The figure shows three views and two pictorial views of one solid part (mm, origin at its lowest corner). Answer the questions. A direction names the side the tool comes from. Give positions to 0.01 mm unless a question says otherwise; leave off trailing zeros. Write each loop counter-clockwise with the first axis right and the second up, starting at its lowest first coordinate (ties: lowest second). Pieces come first, ordered by that corner, then holes. Notation, with made-up numbers: (19, 63.25) -> (36, 63.25) arc R10 cw to (36, 73.25) -> close; hole circle Ø1 at (49.25, 23.25). An arc over 180 degrees is marked (long way). Use a Markdown table: item, result.
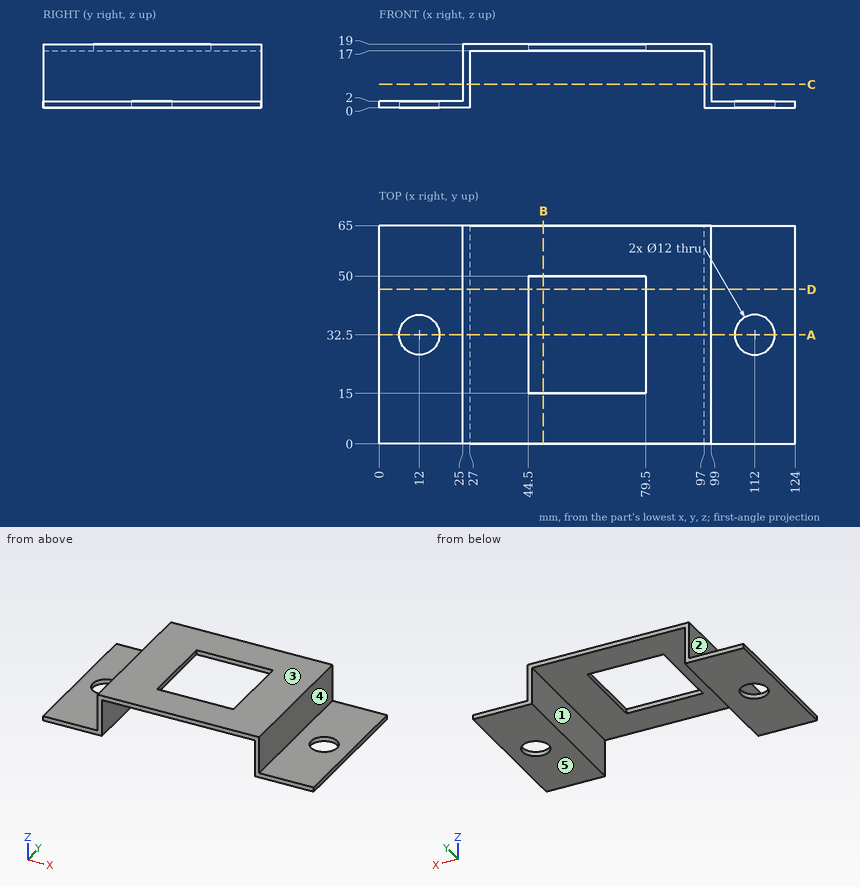
Item 1: A cutting plane is placed at C-C (z = 7). Give the vertices of the cut face in (x, y).
Return value:
| item | result |
|---|---|
| outline | (25, 0) -> (27, 0) -> (27, 65) -> (25, 65) -> close; (97, 0) -> (99, 0) -> (99, 65) -> (97, 65) -> close |
Item 2: Each of these flat-tipped pins is pushed along its axis until it touches: P1, Ø8.5, axis at y = 31, z = 6.5, coming from the +X side; P2, Ø4, axis at x = 20.5, y = 27, coming from the +Z side; P3, Ø1, axis at y = 56, z = 11.5, coming from the -X side; P4, Ø11, axis at x = 112, y = 32.5, coming from the +Z side. Where does it stop, or does it pass through?
Return value:
| item | result |
|---|---|
| P1 | x = 99 |
| P2 | z = 2 |
| P3 | x = 25 |
| P4 | through |
Item 3: A cutting plane is placed at B-B (x = 49). Give the vertices of the cut face in (y, z).
Return value:
| item | result |
|---|---|
| outline | (0, 17) -> (15, 17) -> (15, 19) -> (0, 19) -> close; (50, 17) -> (65, 17) -> (65, 19) -> (50, 19) -> close |
Item 4: A tool of negligible diameter and unlimited length cuts with its end or side. For the marked faces 1, 2, 3, 4 and 5, from which of +Z, -Z, +X, -X, +Y, -Y can it reach the whole face along a straight path? Write none if from no direction.
Return value:
| item | result |
|---|---|
| face 1 | -Z, +Y, -Y |
| face 2 | +Z, -X, +Y, -Y |
| face 3 | +Z, +X, -X, +Y, -Y |
| face 4 | +Z, +X, +Y, -Y |
| face 5 | -Z, +X, -X, +Y, -Y |
Item 5: A cutting plane is placed at A-A (y = 32.5). Give the vertices of the cut face in (x, z).
Return value:
| item | result |
|---|---|
| outline | (0, 0) -> (6, 0) -> (6, 2) -> (0, 2) -> close; (18, 0) -> (27, 0) -> (27, 17) -> (44.5, 17) -> (44.5, 19) -> (25, 19) -> (25, 2) -> (18, 2) -> close; (79.5, 17) -> (97, 17) -> (97, 0) -> (106, 0) -> (106, 2) -> (99, 2) -> (99, 19) -> (79.5, 19) -> close; (118, 0) -> (124, 0) -> (124, 2) -> (118, 2) -> close |
Item 6: A cutting plane is placed at D-D (y = 46). Give the vertices of the cut face in (x, z).
Return value:
| item | result |
|---|---|
| outline | (0, 0) -> (27, 0) -> (27, 17) -> (44.5, 17) -> (44.5, 19) -> (25, 19) -> (25, 2) -> (0, 2) -> close; (79.5, 17) -> (97, 17) -> (97, 0) -> (124, 0) -> (124, 2) -> (99, 2) -> (99, 19) -> (79.5, 19) -> close |
Item 7: Straight lines are drawn through the part: line 1 along Y through (x, z) = (12, 1.15); line 2 along X through (y, z) = (12, 15); line 3 along Z through (x, y) = (8.5, 43.5). For each, find the intervals that lie inside material, in ascending order. Write a range as [from, to].
Return value:
| item | result |
|---|---|
| line 1 | [0, 26.5], [38.5, 65] |
| line 2 | [25, 27], [97, 99] |
| line 3 | [0, 2] |
